Autodesk Inventor part; units mm, degrees
ref_plane "YZ Plane" through (0, 0, 0) normal (1, 0, 0) x (0, 1, 0)
ref_plane "XZ Plane" through (0, 0, 0) normal (0, 1, 0) x (-1, 0, 0)
ref_plane "XY Plane" through (0, 0, 0) normal (0, 0, 1) x (1, 0, 0)
sketch "Sketch1" plane through (0, 0, 0) normal (0, 0, 1) x (1, 0, 0)
  line L0 (-300, -140) -> (120, -140)
  line L1 (120, -140) -> (120, 140)
  line L2 (120, 140) -> (-300, 140)
  line L3 (-300, 140) -> (-300, -140)
  point P0 (0, 0)
  dimension "d0" = 420
  dimension "d1" = 280
  dimension "d36" = 300
sketch "Sketch4" plane through (0, 0, 0) normal (0, 0, 1) x (1, 0, 0)
  line L0 (-273, -1) -> (-260.5, -1)
  line L1 (-148, -1) -> (-148, -13.5)
  line L2 (-148, -126) -> (-160.5, -126)
  line L3 (-273, -126) -> (-273, -113.5)
  line L4 (-273, -13.5) -> (-260.5, -1)
  line L5 (-160.5, -1) -> (-148, -13.5)
  line L6 (-148, -113.5) -> (-160.5, -126)
  line L7 (-260.5, -126) -> (-273, -113.5)
  line L8 (-260.5, -1) -> (-160.5, -1)
  line L9 (-273, -13.5) -> (-273, -1)
  line L10 (-160.5, -1) -> (-148, -1)
  line L11 (-148, -13.5) -> (-148, -113.5)
  line L12 (-160.5, -126) -> (-260.5, -126)
  line L13 (-148, -113.5) -> (-148, -126)
  line L14 (-260.5, -126) -> (-273, -126)
  line L15 (-273, -113.5) -> (-273, -13.5)
  line L16 (-300, -140) -> (120, -140)
  line L17 (-300, 140) -> (-300, -140)
  point P0 (0, 0)
  dimension "d6" = 125
  dimension "d7" = 125
  dimension "d8" = 12.5
  dimension "d9" = 12.5
  dimension "d10" = 12.5
  dimension "d11" = 12.5
  dimension "d12" = 12.5
  dimension "d13" = 12.5
  dimension "d14" = 12.5
  dimension "d15" = 12.5
  dimension "d22" = 14
  dimension "d23" = 27
sketch "Sketch5" plane through (0, 0, 0) normal (0, 0, 1) x (1, 0, 0)
  line L0 (-273, -13.5) -> (-260.5, -1)
  line L1 (-260.5, -1) -> (-160.5, -1)
  line L2 (-160.5, -1) -> (-148, -13.5)
  line L3 (-148, -13.5) -> (-148, -113.5)
  line L4 (-160.5, -126) -> (-260.5, -126)
  line L5 (-148, -113.5) -> (-160.5, -126)
  line L6 (-260.5, -126) -> (-273, -113.5)
  line L7 (-273, -113.5) -> (-273, -13.5)
  point P0 (0, 0)
boundary_patch "Boundary Patch3"
pattern_linear "Rectangular Pattern1" count 3 spacing 127 along (1, 0, 0) count 2 spacing 127 along (0, 1, 0) of "Boundary Patch3"
sketch "Sketch6" plane through (0, 0, 0) normal (0, 0, 1) x (1, 0, 0)
  line L0 (120, 140) -> (-300, 140)
  line L1 (-300, 140) -> (-300, -140)
  line L2 (-300, -140) -> (120, -140)
  line L3 (120, -140) -> (120, 140)
  line L4 (-260.5, 126) -> (-160.5, 126)
  line L5 (-133.5, 126) -> (-33.5, 126)
  line L6 (-146, 113.5) -> (-133.5, 126)
  line L7 (-160.5, 126) -> (-148, 113.5)
  line L8 (-273, 13.5) -> (-273, 113.5)
  line L9 (-273, 113.5) -> (-260.5, 126)
  line L10 (-260.5, 1) -> (-273, 13.5)
  line L11 (-160.5, 1) -> (-260.5, 1)
  line L12 (-148, 113.5) -> (-148, 13.5)
  line L13 (-148, 13.5) -> (-160.5, 1)
  line L14 (-133.5, 1) -> (-146, 13.5)
  line L15 (-146, 13.5) -> (-146, 113.5)
  line L16 (-21, 113.5) -> (-21, 13.5)
  line L17 (-19, 13.5) -> (-19, 113.5)
  line L18 (-33.5, 126) -> (-21, 113.5)
  line L19 (-19, 113.5) -> (-6.5, 126)
  line L20 (-6.5, 126) -> (93.5, 126)
  line L21 (93.5, 126) -> (106, 113.5)
  line L22 (106, 113.5) -> (106, 13.5)
  line L23 (-273, -113.5) -> (-273, -13.5)
  line L24 (-273, -13.5) -> (-260.5, -1)
  line L25 (-160.5, -1) -> (-148, -13.5)
  line L26 (-260.5, -1) -> (-160.5, -1)
  line L27 (-146, -13.5) -> (-133.5, -1)
  line L28 (-33.5, -1) -> (-21, -13.5)
  line L29 (-133.5, -1) -> (-33.5, -1)
  line L30 (-33.5, 1) -> (-133.5, 1)
  line L31 (-21, 13.5) -> (-33.5, 1)
  line L32 (106, 13.5) -> (93.5, 1)
  line L33 (-6.5, 1) -> (-19, 13.5)
  line L34 (93.5, 1) -> (-6.5, 1)
  line L35 (-6.5, -1) -> (93.5, -1)
  line L36 (-19, -13.5) -> (-6.5, -1)
  line L37 (93.5, -1) -> (106, -13.5)
  line L38 (-160.5, -126) -> (-260.5, -126)
  line L39 (-148, -13.5) -> (-148, -113.5)
  line L40 (-146, -113.5) -> (-146, -13.5)
  line L41 (-21, -13.5) -> (-21, -113.5)
  line L42 (-19, -113.5) -> (-19, -13.5)
  line L43 (106, -13.5) -> (106, -113.5)
  line L44 (106, -113.5) -> (93.5, -126)
  line L45 (93.5, -126) -> (-6.5, -126)
  line L46 (-6.5, -126) -> (-19, -113.5)
  line L47 (-21, -113.5) -> (-33.5, -126)
  line L48 (-33.5, -126) -> (-133.5, -126)
  line L49 (-133.5, -126) -> (-146, -113.5)
  line L50 (-148, -113.5) -> (-160.5, -126)
  line L51 (-260.5, -126) -> (-273, -113.5)
  point P0 (0, 0)
sketch "Sketch9" plane through (0, 0, 0) normal (0, 0, 1) x (1, 0, 0)
  line L0 (-260.5, 126) -> (-160.5, 126)
  line L1 (-160.5, 126) -> (-148, 113.5)
  line L2 (-148, 113.5) -> (-148, 13.5)
  line L3 (-273, 13.5) -> (-273, 113.5)
  line L4 (-273, 113.5) -> (-260.5, 126)
  line L5 (-160.5, 1) -> (-260.5, 1)
  line L6 (-260.5, 1) -> (-273, 13.5)
  line L7 (-273, -13.5) -> (-260.5, -1)
  line L8 (-260.5, -1) -> (-160.5, -1)
  line L9 (-273, -113.5) -> (-273, -13.5)
  line L10 (-160.5, -1) -> (-148, -13.5)
  line L11 (-148, -13.5) -> (-148, -113.5)
  line L12 (-148, 13.5) -> (-160.5, 1)
  line L13 (-133.5, 1) -> (-146, 13.5)
  line L14 (-146, -13.5) -> (-133.5, -1)
  line L15 (-146, -113.5) -> (-146, -13.5)
  line L16 (-146, 13.5) -> (-146, 113.5)
  line L17 (-133.5, 126) -> (-33.5, 126)
  line L18 (-146, 113.5) -> (-133.5, 126)
  line L19 (-33.5, 126) -> (-21, 113.5)
  line L20 (-21, 113.5) -> (-21, 13.5)
  line L21 (-21, 13.5) -> (-33.5, 1)
  line L22 (-33.5, 1) -> (-133.5, 1)
  line L23 (-133.5, -1) -> (-33.5, -1)
  line L24 (-33.5, -126) -> (-133.5, -126)
  line L25 (-160.5, -126) -> (-260.5, -126)
  line L26 (-260.5, -126) -> (-273, -113.5)
  line L27 (-148, -113.5) -> (-160.5, -126)
  line L28 (-21, -113.5) -> (-33.5, -126)
  line L29 (-133.5, -126) -> (-146, -113.5)
  line L30 (-33.5, -1) -> (-21, -13.5)
  line L31 (-6.5, 1) -> (-19, 13.5)
  line L32 (106, 13.5) -> (93.5, 1)
  line L33 (93.5, -1) -> (106, -13.5)
  line L34 (106, 113.5) -> (106, 13.5)
  line L35 (93.5, 1) -> (-6.5, 1)
  line L36 (-6.5, -1) -> (93.5, -1)
  line L37 (93.5, -126) -> (-6.5, -126)
  line L38 (-19, -113.5) -> (-19, -13.5)
  line L39 (-21, -13.5) -> (-21, -113.5)
  line L40 (106, -13.5) -> (106, -113.5)
  line L41 (-19, -13.5) -> (-6.5, -1)
  line L42 (-19, 13.5) -> (-19, 113.5)
  line L43 (-6.5, 126) -> (93.5, 126)
  line L44 (-19, 113.5) -> (-6.5, 126)
  line L45 (93.5, 126) -> (106, 113.5)
  line L46 (106, -113.5) -> (93.5, -126)
  line L47 (-6.5, -126) -> (-19, -113.5)
extrude "Extrusion4" add sketch "Sketch6" against normal blind 2
extrude "Extrusion6" add sketch "Sketch9" against normal blind 1.9
equation "\"d9\" = d8"
equation "\"d10\" = d9"
equation "\"d11\" = d10"
equation "\"d12\" = d11"
equation "\"d13\" = d12"
equation "\"d14\" = d13"
equation "\"d15\" = d8"
properties part number "solar1" material "Aluminum 6061-AHC"
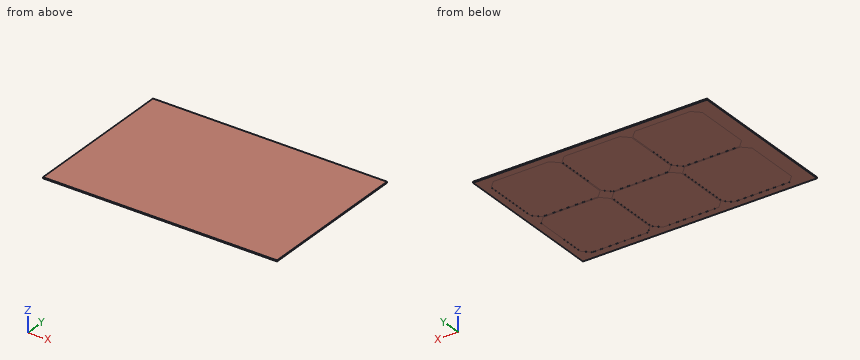
Build history of the part. All positions in model axes, mm. Give positions to 0.01 mm unless a question says otherwise; leave off trailing zeros. Loops run counter-clockwise (first coordinate to the right, second up) from the corner with the lowest first, then second, coordinate; pieces in that order, holes last. Notation, with made-up numbers: (-33.5, -35) - (-7.5, -35) arc R23 cw to (-7.5, -9) - close; hole circle Ø11 at (26.5, 30.5). An arc over 180 degrees is marked (long way). Write item = value, one per line. Start each with the question number.
1) Band-saw the part on A-A on x = -217. Give the cut face in (y, z).
2) Probe probe 1 along Z at (x, y) = (34, -105.5). List the from-to ranges inside material, lowest first. Write a range as from..to.
3) Drop flat-ended pins along their axis: pin 1 Ø12 at (x, y) = (-107.5, 3) entering from -Z; pin 2 Ø5 at (x, y) = (-54, 76.5) entering from -Z. Give the stop position or say it passes through.
4) Band-saw the part on B-B on y = 68.5. Give the cut face in (x, z).
Final values:
q1.outline = (-140, -2) - (-126, -2) - (-126, -1.9) - (-1, -1.9) - (-1, -2) - (1, -2) - (1, -1.9) - (126, -1.9) - (126, -2) - (140, -2) - (140, 0) - (-140, 0) - close
q2.probe_1 = -1.9..0
q3.pin_1 = -2
q3.pin_2 = -1.9
q4.outline = (-300, -2) - (-273, -2) - (-273, -1.9) - (-148, -1.9) - (-148, -2) - (-146, -2) - (-146, -1.9) - (-21, -1.9) - (-21, -2) - (-19, -2) - (-19, -1.9) - (106, -1.9) - (106, -2) - (120, -2) - (120, 0) - (-300, 0) - close
